```python
from build123d import *

# Parameters (mm, degrees)
SKETCH1_W           = 20
SKETCH1_H           = 10
SKETCH1_R           = 3
SKETCH1_R_2         = 1.5
BOSS_EXTRUDE1_DEPTH = 3
SKETCH2_W           = 10
SKETCH2_H           = 10
BOSS_EXTRUDE2_DEPTH = 2
SKETCH3_W           = 10
SKETCH3_H           = 10
BOSS_EXTRUDE3_DEPTH = 1
FILLET1_R           = 4
FILLET2_START       = -5
FILLET2_DEPTH       = 12
FILLET2_START_2     = -3.811659193
FILLET2_2_DEPTH     = 10
FILLET3_R           = 1


with BuildPart() as part:
    # Sketch1 → Boss-Extrude1 (new body)
    with BuildSketch(Plane.XY):
        with Locations((1.143497758, 1.188340807)):
            Rectangle(SKETCH1_W, SKETCH1_H)
        with Locations((-4.356502242, 1.188340807)):
            Circle(SKETCH1_R, mode=Mode.SUBTRACT)
        with Locations((6.643497758, 1.188340807)):
            Circle(SKETCH1_R, mode=Mode.SUBTRACT)
        with Locations((1.143497758, 1.188340807)):
            Circle(SKETCH1_R_2, mode=Mode.SUBTRACT)
    extrude(amount=BOSS_EXTRUDE1_DEPTH)

    # Sketch2 → Boss-Extrude2 (add)
    with BuildSketch(Plane.XY.offset(3)):
        with Locations((16.143497758, 1.188340807)):
            Rectangle(SKETCH2_W, SKETCH2_H)
    extrude(amount=-BOSS_EXTRUDE2_DEPTH)

    # Sketch3 → Boss-Extrude3 (add)
    with BuildSketch(Plane.XY.offset(3)):
        with Locations((26.143497758, 1.188340807)):
            Rectangle(SKETCH3_W, SKETCH3_H)
    extrude(amount=-BOSS_EXTRUDE3_DEPTH)


with BuildPart() as body_2:
    # Mirror3: mirrored copy
    add(part.part.mirror(Plane(origin=(26.143497758, 0, 0), x_dir=(0, 0, 1), z_dir=(1, 0, 0))))


with BuildPart() as part_1:
    add(part.part)

    # Combine1: union body 2
    add(body_2.part)

    # Fillet1
    fillet1_edges = [part_1.edges().sort_by_distance(p)[0] for p in [
        (61.143497758, -3.811659193, 1.5),
        (-8.856502242, -3.811659193, 1.5),
    ]]
    fillet(fillet1_edges, radius=FILLET1_R)

    # Fillet2: read off the stored shape, not the designer's step
    # Fillet2 outline → Fillet2 (cut)
    with BuildSketch(Plane(origin=(0, 0, 0), x_dir=(1, 0, 0), z_dir=(0, 1, 0)).offset(FILLET2_START)):
        with BuildLine():
            Line((31.143497758, -1), (31.143497758, -2))
            ThreePointArc((31.143497758, -2), (31.436390977, -1.292893219), (32.143497758, -1))
            Line((32.143497758, -1), (31.143497758, -1))
        make_face()
    extrude(amount=FILLET2_DEPTH, mode=Mode.SUBTRACT)

    # Fillet2 2 outline → Fillet2 2 (add)
    with BuildSketch(Plane(origin=(0, 0, 0), x_dir=(1, 0, 0), z_dir=(0, 1, 0)).offset(FILLET2_START_2)):
        with BuildLine():
            ThreePointArc((41.143497758, 0), (40.850604539, -0.707106781), (40.143497758, -1))
            Line((40.143497758, -1), (41.143497758, -1))
            Line((41.143497758, -1), (41.143497758, 0))
        make_face()
    extrude(amount=FILLET2_2_DEPTH)

    # Fillet3
    # the kernel refuses this fillet: 1 mm, written as the material it takes off along each edge
    with BuildSketch(Plane(origin=(-4.356502242, 1.188340807, 0), x_dir=(1, 0, 0), z_dir=(0, -1, 0))) as fillet3_piece_1:
        with BuildLine():
            CenterArc((3 + FILLET3_R, FILLET3_R), FILLET3_R, 180, 90)
            Line((3, FILLET3_R), (3, 0))
            Line((3, 0), (3 + FILLET3_R, 0))
        make_face()
    revolve(axis=Axis((-4.356502242, 1.188340807, 0), (0, 0, 1)), mode=Mode.SUBTRACT)
    with BuildSketch(Plane(origin=(6.643497758, 1.188340807, 0), x_dir=(1, 0, 0), z_dir=(0, -1, 0))) as fillet3_piece_2:
        with BuildLine():
            CenterArc((3 + FILLET3_R, FILLET3_R), FILLET3_R, 180, 90)
            Line((3, FILLET3_R), (3, 0))
            Line((3, 0), (3 + FILLET3_R, 0))
        make_face()
    revolve(axis=Axis((6.643497758, 1.188340807, 0), (0, 0, 1)), mode=Mode.SUBTRACT)
    with BuildSketch(Plane(origin=(1.143497758, 1.188340807, 0), x_dir=(1, 0, 0), z_dir=(0, -1, 0))) as fillet3_piece_3:
        with BuildLine():
            CenterArc((1.5 + FILLET3_R, FILLET3_R), FILLET3_R, 180, 90)
            Line((1.5, FILLET3_R), (1.5, 0))
            Line((1.5, 0), (1.5 + FILLET3_R, 0))
        make_face()
    revolve(axis=Axis((1.143497758, 1.188340807, 0), (0, 0, 1)), mode=Mode.SUBTRACT)


solid = part_1.part
```
Can you work these out from the model? Positions are in its coordinate system, mm. A direction names the side the tool comes from. Round coordinates to 2 decimals unless told otherwise and drop trailing zeros. Order: outer loops, then holes, each group sorted by start corner. A loop starts at its lowest first (then second) coordinate and runs counter-clockwise, first axis right, second up.
(1) If we section it at A-A (x = 50.5): Please give me the cut outline in (y, z), plus the area to 3 significant figures.
Results are:
outline: (-3.81, 0) - (-0.17, 0) - (-0.17, 3) - (-3.81, 3) - close; (2.54, 0) - (6.19, 0) - (6.19, 3) - (2.54, 3) - close
area: 21.9 mm2
(2) We'd pull the mould along Y, two halves only. Please class faces 3 (the face through (59.94, -2.67, 1.52)), 4 (the face through (-7.354, 1.32, 1.986)), 5 (the face through (26, 1, 2)), 6 (the face through (25.7, 6.188, 2.5)): +Y half, -Y half, draft (parallel to the pull), parting line (faces both ways), or undercut.
Results are:
face 3: -Y half
face 4: undercut
face 5: draft
face 6: +Y half
(3) I'm going to push flat-ended pins straight in: pin 1 (5 mm diameter, centred on x = 26.5, y = 1.5, fed in from -Z); pin 2 (0.8 mm diameter, centred on y = 0, z = 1.5, fed in from +X); pin 3 (5 mm diameter, centred on x = 16, y = 0.5, fed in from -Z); pin 4 (1.8 mm diameter, centred on x = 51.14, y = 1.19, fed in from -Z). Where does each tip first touch, or does it pass through?
Results are:
pin 1: stops at z = 2
pin 2: stops at x = 61.14
pin 3: stops at z = 1
pin 4: passes through
(4) If we section it at C-C (x = 37): Please give me the cut outline in (y, z), plus the area to 3 significant figures.
Results are:
outline: (-3.81, 1) - (6.19, 1) - (6.19, 3) - (-3.81, 3) - close
area: 20.0 mm2
(5) If I drill on L1, parallel to Y at x = 6.5, z = 1.8; L2, parallel to X at y = 5, z = 1.15; L3, parallel to Y at x = 51.5, z = 0.25, over which ranges is the centre line in solid material (lowest first)?
Results are:
L1: y = -3.81 to -1.81, 4.18 to 6.19
L2: x = -8.86 to 21.14, 31.62 to 61.14
L3: y = -3.81 to -0.27, 2.65 to 6.19
(6) On a 3-axis mill with a long thin cutter (end or side, diameter ignored), from which of +Z, -Z, +X, -X, +Y, -Y can I reach the whole of each face in a straight line? I mean faces 1 (the face through (-8.857, 3, 1)), 2 (the face through (16, 1, 1)). Say none if no direction works.
Results are:
face 1: +Z, -Z, -X, +Y, -Y
face 2: -Z, +Y, -Y
(7) If we section it at B-B (x = 23): Please give me the cut outline in (y, z).
Results are:
outline: (-3.81, 2) - (6.19, 2) - (6.19, 3) - (-3.81, 3) - close
